from build123d import *

# Parameters (mm, degrees)
F0_R     = 15.875
F1_DEPTH = 25.4
F2_W     = 43.094914
F2_H     = 19.034712
F3_DEPTH = 19.05
F4_R     = 1.8288
F5_DEPTH = 6.351
F6_R     = 12.7
F7_DEPTH = 12.7
F8_R     = 3.175
F9_DEPTH = 23.0124


with BuildPart() as f1:
    # F0 (on Right) → F1 (new body)
    with BuildSketch(Plane.YZ):
        Circle(F0_R)
    extrude(amount=F1_DEPTH)

    # F2 (on face) → F3 (cut)
    with BuildSketch(Plane.YZ.offset(25.4)):
        with Locations((0.400271, -9.517356)):
            Rectangle(F2_W, F2_H)
    extrude(amount=-F3_DEPTH, mode=Mode.SUBTRACT)

    # F4 (on face) → F5 (cut, through all)
    with BuildSketch(Plane.YZ.offset(6.35)):
        Circle(F4_R)
    extrude(amount=-F5_DEPTH, mode=Mode.SUBTRACT)

    # F6 (on face) → F7 (cut)
    with BuildSketch(Plane.YZ.offset(25.4)):
        Circle(F6_R)
    extrude(amount=-F7_DEPTH, mode=Mode.SUBTRACT)

    # F8 (on face) → F9 (cut)
    with BuildSketch(Plane.YZ.offset(25.4)):
        Circle(F8_R)
    extrude(amount=-F9_DEPTH, mode=Mode.SUBTRACT)


solid = f1.part
The listing builds one solid part. Answer for the finished solid, in the listing's coordinates (mm). A direction names the side the tool comes from. Give positions to 0.01 mm unless a question says otherwise; leave off trailing zeros. Loops run counter-clockwise (first coordinate to the right, second up) from the corner with the lowest first, then second, coordinate; pieces in that order, holes last. Notation, with made-up numbers: (-28.75, -39) - (-21.75, -39) arc R22 cw to (-21.75, -4) - close; hole circle Ø9 at (44, -26). An arc over 180 degrees is marked (long way). Write each question's results on one line, items separated by ' | '.
1. Consider probe 1 along Z at (x, y) = (1.85, 0) (3 decimals); probe 2 along Z at (x, y) = (4, 0) (3 decimals); probe 3 along X at (y, z) = (-1, -6.5). Determine where each line is inside the solid, lowest interval first. Write a range as from..to.
Resolved:
probe 1: z = -15.875..-1.829, 1.829..15.875 | probe 2: z = -15.875..-3.175, 3.175..15.875 | probe 3: x = 0..6.35
2. Find section B-B, the plane z = -1. Write down the section's boundary in (x, y).
Resolved:
outline: (0, -15.84) - (6.35, -15.84) - (6.35, -3.01) - (2.39, -3.01) - (2.39, -1.53) - (0, -1.53) - close; (0, 1.53) - (2.39, 1.53) - (2.39, 3.01) - (6.35, 3.01) - (6.35, 15.84) - (0, 15.84) - close
3. Which of the six approach directions +Z, -Z, +X, -X, +Y, -Y give full straight-line access (tool end or side, diameter ignored) to faces 1 (the face through (12, 11, 0)), 2 (the face through (25.4, -1, 13)), 3 (the face through (6.47, -0.41, 3.15)), 4 (the face through (0, 3, 0)), 5 (the face through (12.7, 0, 6))?
Resolved:
face 1: -Z, +X, +Y, -Y | face 2: +Z, -Z, +X, +Y, -Y | face 3: +X | face 4: +Z, -Z, -X, +Y, -Y | face 5: -Z, +X
4. Find section D-D, the plane z = 11.5. Write down the section's boundary in (x, y), then the cut area to 3 significant figures.
Resolved:
outline: (0, -10.94) - (25.4, -10.94) - (25.4, -5.39) - (12.7, -5.39) - (12.7, 5.39) - (25.4, 5.39) - (25.4, 10.94) - (0, 10.94) - close | area: 419 mm^2
5. For a pull along Z with two mould halves and no side action, classify faces 6 (the face through (2.388, 1.4, -1.4)), 7 (the face through (6.35, 0, -6)), 8 (the face through (9.7, -2.07, 15.74)), 9 (the face through (19.139, 0.279, 12.697)) as +Z half, -Z half, draft (parallel to the pull), parting line (faces both ways), or undercut.
Resolved:
face 6: undercut | face 7: draft | face 8: parting line | face 9: -Z half
6. Find section A-A, the plane y = 0. Write down the section's boundary in (x, z) (3 decimals), then the cut area to 3 significant figures.
Resolved:
outline: (0, -15.875) - (6.35, -15.875) - (6.35, -3.175) - (2.388, -3.175) - (2.388, -1.829) - (0, -1.829) - close; (0, 1.829) - (2.388, 1.829) - (2.388, 3.175) - (12.7, 3.175) - (12.7, 12.7) - (25.4, 12.7) - (25.4, 15.875) - (0, 15.875) - close | area: 289 mm^2
7. Find section C-C, the plane x = 3.5. Write down the section's boundary in (y, z) (3 decimals), then the cut area to 3 significant figures.
Resolved:
outline: circle Ø31.75 at (0, 0); hole circle Ø6.35 at (0, 0) | area: 760 mm^2
8. Flat-ended cylindrical pins translate along their axes: P1, Ø1, axis at x = 18.5, y = 1, coming from the +Z side; P2, Ø3.5, axis at y = 0, z = 0, coming from the -X side; P3, Ø3, axis at x = 22, y = 10, coming from the -Z side; P4, Ø6.5, axis at y = -1.5, z = 4.5, coming from the +X side. Find the tip coordinate at first contact, or state that the pin passes through.
Resolved:
P1: stops at z = 15.87 | P2: passes through | P3: stops at z = 5.39 | P4: stops at x = 12.7
